```python
from build123d import *

# Parameters (mm, degrees)
SKETCH_1_R      = 2.6
EXTRUDE_1_DEPTH = 22


with BuildPart() as part:
    # 草图1 → 凸台-拉伸1 (new body)
    with BuildSketch(Plane.XY):
        with BuildLine():
            Line((23.847340939, 22.540535696), (25.426595378, -0.670423871))
            add(Edge.make_bspline(
                [(-45.075558205, -69.325666874), (-42.754308832, -67.574416213), (-40.451669282, -65.798512541), (-32.294309234, -59.368468615), (-26.546100007, -54.578255108), (-15.345136182, -44.664021117), (-9.895646996, -39.536602487), (0.681335287, -28.95909339), (5.808236447, -23.509575428), (15.763503709, -12.344368812), (20.592346629, -6.630730984), (25.344702666, -0.771444989), (25.385653413, -0.720937959), (25.426595378, -0.670423871)],
                knots=[0.201401882, 0.201401882, 0.201401882, 0.201401882, 0.25, 0.25, 0.375, 0.375, 0.5, 0.5, 0.625, 0.625, 0.75, 0.75, 0.751086715, 0.751086715, 0.751086715, 0.751086715], degree=3))
            Line((-45.075558205, -69.325666874), (-46.403218206, -49.812495445))
            add(Edge.make_bspline(
                [(23.847340939, 22.540535696), (23.64915353, 22.233291982), (23.450485571, 21.926356885), (19.302193238, 15.53957719), (15.159702589, 9.585176101), (8.596754946, 0.915295883), (6.3513379, -1.931247492), (1.744627248, -7.528266651), (-0.617237974, -10.279137899), (-5.445852464, -15.685888726), (-7.913195994, -18.342470215), (-11.674958808, -22.267979722), (-12.938982587, -23.567073503), (-15.483103595, -26.149104874), (-16.762445153, -27.432760042), (-20.640021965, -31.243741747), (-23.278577451, -33.732226441), (-28.749348744, -38.491244165), (-31.58193298, -40.761476786), (-37.50215526, -44.948079537), (-40.590801141, -46.863006315), (-44.66457019, -48.977283832), (-45.52963212, -49.403999667), (-46.403218206, -49.812495445)],
                knots=[0.243696274, 0.243696274, 0.243696274, 0.243696274, 0.25, 0.25, 0.375, 0.375, 0.4375, 0.4375, 0.5, 0.5, 0.5625, 0.5625, 0.59375, 0.59375, 0.625, 0.625, 0.6875, 0.6875, 0.75, 0.75, 0.8125, 0.8125, 0.829122533, 0.829122533, 0.829122533, 0.829122533], degree=3))
        make_face()
        with Locations((-36.167886121, -52.931465967)):
            Circle(SKETCH_1_R, mode=Mode.SUBTRACT)
        with Locations((15.466595378, -1.598123556)):
            Circle(SKETCH_1_R, mode=Mode.SUBTRACT)
    extrude(amount=EXTRUDE_1_DEPTH)


solid = part.part
```
Here's how the part is built. I have some questions about the finished solid (model axes, mm). Round coordinates to 2 decimals unless told otherwise and drop trailing zeros. Answer as CSV lines item,"result". Start each with the question number.
1. I need wall thicknesses on probe 1 along Y at (x, z) = (15, 8.5); probe 2 along X at (y, z) = (9, 2.5); probe 3 along X at (y, z) = (-62.5, 15.25). Which ranges of each line are inside material? Lowest first, please.
2. Suppose I cut it at A-A on z = 11. Count the separate pieces of the cut face and the enclosed holes in it, then the cut area to 3 significant figures.
3. I'm going to push flat-ended pins straight in: pin 1 Ø5 at (x, y) = (-20, -41.5) entering from -Z; pin 2 Ø12 at (y, z) = (-22, 8) entering from +X; pin 3 Ø12 at (y, z) = (-5.5, 11.5) entering from +X; pin 4 Ø3 at (y, z) = (-56, 17.5) entering from -X. Where does each tip first touch, or does it pass through?
4. Thinking about a two-plate mould opening in Y: for faces 1 (the flat face through (-10, -27, 22)), 2 (the flat face through (24.626, 11.098, 10.846)), 3 (the cylindrical face through (-36.506, -50.354, 10.846)), which applies, released by +Y, released by -Y, zero draft, split by the parting line, or undercut?
Check result:
1,probe 1,"y = -13.13 to -4.16, 0.96 to 9.53"
1,probe 2,"x = 14.62 to 24.77"
1,probe 3,"x = -45.54 to -36.28"
2,separate pieces,"1"
2,enclosed holes,"2"
2,area,"1,360 mm2"
3,pin 1,"stops at z = 0"
3,pin 2,"stops at x = 12.49"
3,pin 3,"stops at x = 25.43"
3,pin 4,"stops at x = -46.08"
4,face 1,"zero draft"
4,face 2,"released by +Y"
4,face 3,"undercut"
